from build123d import *

# Parameters (mm, degrees)
SKETCH1_W             = 45.55
SKETCH1_H             = 50.8
BOSS_EXTRUDE1_DEPTH   = 6.35
SKETCH2_W             = 15
SKETCH2_H             = 6.35
SKETCH2_W_2           = 15.55
CUT_EXTRUDE1_DEPTH    = 6.35
F_6_CLEARANCE_HOLE1_D = 3.6576


with BuildPart() as part:
    # Sketch1 → Boss-Extrude1 (new body)
    with BuildSketch(Plane.XY):
        Rectangle(SKETCH1_W, SKETCH1_H)
    extrude(amount=BOSS_EXTRUDE1_DEPTH)

    # Sketch2 → Cut-Extrude1 (cut)
    with BuildSketch(Plane.XY.offset(6.35)):
        with Locations((-15.275, -22.225)):
            Rectangle(SKETCH2_W, SKETCH2_H)
        with Locations((15, -22.225)):
            Rectangle(SKETCH2_W_2, SKETCH2_H)
    cut_extrude1 = extrude(amount=-CUT_EXTRUDE1_DEPTH, mode=Mode.SUBTRACT)

    # #6 Clearance Hole1 (through all)
    with Locations(Plane.XY.offset(6.35)):
        with Locations((-0.275, -22.225)):
            f_6_clearance_hole1 = Hole(F_6_CLEARANCE_HOLE1_D / 2)

    # Mirror1: Cut-Extrude1, #6 Clearance Hole1 across plane
    add(cut_extrude1.mirror(Plane.ZX), mode=Mode.SUBTRACT)
    add(f_6_clearance_hole1.mirror(Plane.ZX), mode=Mode.SUBTRACT)


solid = part.part
CAD build for the part. Positions are in the model's coordinates, mm. A direction names the side the tool comes from. Give positions to 0.01 mm unless a question says otherwise; leave off trailing zeros. Write each loop counter-clockwise with the first axis right and the second up, starting at its lowest first coordinate (ties: lowest second). Pieces come first, ordered by that corner, then holes. Notation, with made-up numbers: (26.5, -8) - (58.5, -8) arc R25 cw to (58.5, 12) - close; hole circle Ø6 at (4.5, -19). An arc over 180 degrees is marked (long way). Put each result on its own line as item: value.
(1) Pull direction X, two halves, no side cores. Call faces 4 (the flat face through (-7.775, -22, 3)), 5 (the cylindrical face through (0.12, -24.01, 3.13)), 6 (the flat face through (22.775, 0, 3)): released by +X, released by -X, zero draft, split by the parting line, or undercut.
Working result:
face 4: released by -X
face 5: undercut
face 6: released by +X
(2) Saw through at A-A (z = 1.5). List the corners of the cut face in (x, y) (3 decimals), then the cut area to 3 significant figures.
Working result:
outline: (-22.775, -19.05) - (-7.775, -19.05) - (-7.775, -25.4) - (7.225, -25.4) - (7.225, -19.05) - (22.775, -19.05) - (22.775, 19.05) - (7.225, 19.05) - (7.225, 25.4) - (-7.775, 25.4) - (-7.775, 19.05) - (-22.775, 19.05) - close; hole circle Ø3.658 at (-0.275, -22.225); hole circle Ø3.658 at (-0.275, 22.225)
area: 1,900 mm^2
(3) Saw through at B-B (x = -19). List the corners of the cut face in (y, z), then the cut area to 3 significant figures.
Working result:
outline: (-19.05, 0) - (19.05, 0) - (19.05, 6.35) - (-19.05, 6.35) - close
area: 242 mm^2
(4) Drop flat-ended pins along their axis: pin 1 Ø3.5 at (x, y) = (-0.275, 22.225) entering from +Z; pin 2 Ø1.9 at (y, z) = (-23, 4) entering from -X (3 decimals); pin 3 Ø1.9 at (x, z) = (-14, 2.5) entering from -Y; pin 4 Ø2 at (x, y) = (13.5, -13) entering from -Z. Give the stop position or say it passes through.
Working result:
pin 1: through
pin 2: x = -7.775
pin 3: y = -19.05
pin 4: z = 0
(5) Wall check: L1, parallel to Y at x = -0.5, z = 0.75; L2, parallel to Y at x = -10.5, z = 0.5; L3, parallel to X at y = 22.5, z = 6 (3 decimals). Give the ranges that are in metal, low to high.
Working result:
L1: -25.4 to -24.04, -20.41 to 20.41, 24.04 to 25.4
L2: -19.05 to 19.05
L3: -7.775 to -2.083, 1.533 to 7.225
(6) Tool access for faces 1 (the flat face through (15, 19.05, 3)), 2 (the flat face through (15, -19.05, 3)), 3 (the flat face through (-15, -19.05, 3)): list every direction of +Z, -Z, +X, -X, +Y, -Y with a clear straight run to the whole face (end or side of a thin tool).
Working result:
face 1: +Z, -Z, +X, +Y
face 2: +Z, -Z, +X, -Y
face 3: +Z, -Z, -X, -Y
